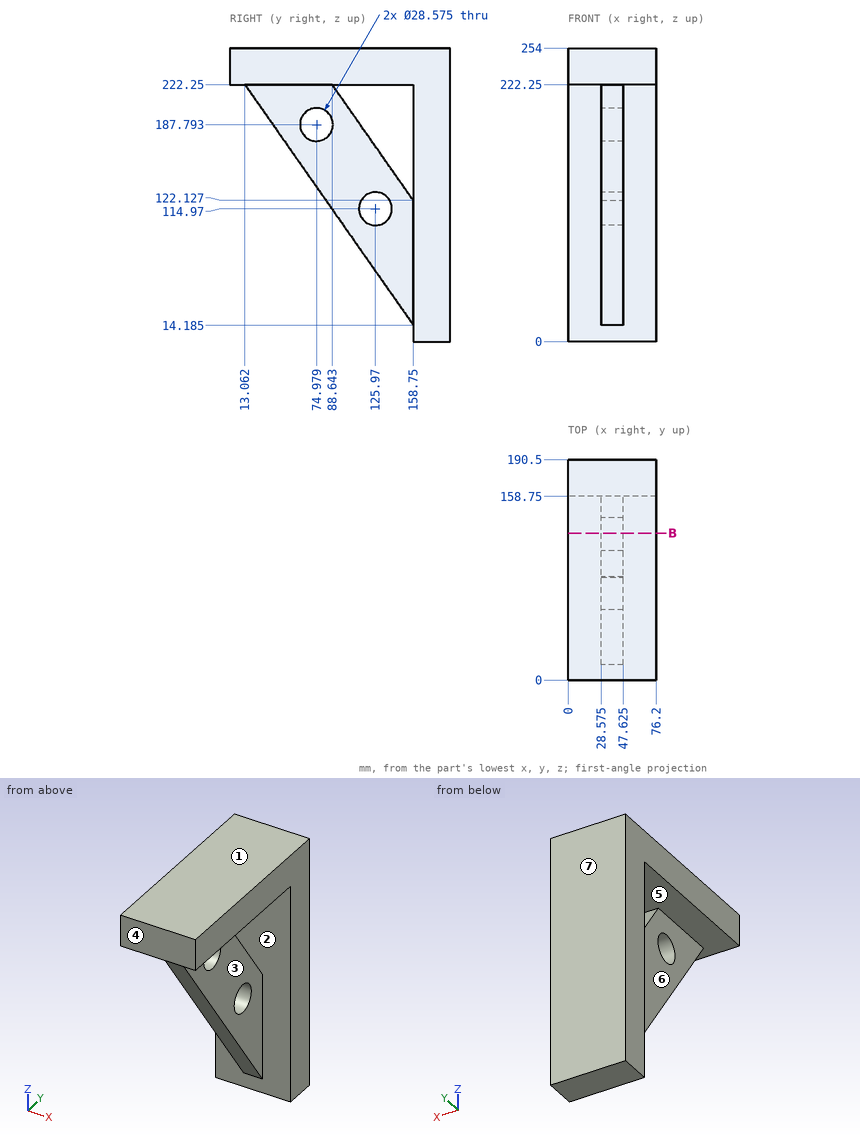
Geometry check sheet. Reference: drawing and pictorial views, mm from the part's lowest x, y, z. A direction names the side the tool comes from. Round coordinates to 2 decimals unless told otherwise and drop trailing zeros. Answer as a JSON object with one key per item and string values.
Q1. Scan lines: line 1 (Y direction, x = 12.5, z = 112.5); line 2 (X direction, y = 116.5, z = 84.5) (1 decimal); line 3 (Z direction, x = 63.5, y = 82.5). Record each from-to range of solid material in increasing order. Write a range as from..to.
Data:
{"line 1": "y = 158.75..190.5", "line 2": "x = 28.6..47.6", "line 3": "z = 222.25..254"}
Q2. Draft check along Y on the marked faces 4, 5, 6 and 7. Enter one of: pulls with the +Y half, pulls with the -Y half, needs draft (parallel to the pull), parting line crosses it, or undercut.
Data:
{"face 4": "pulls with the -Y half", "face 5": "undercut", "face 6": "needs draft", "face 7": "pulls with the +Y half"}
Q3. Section check B-B (y = 127). State how many separate pieces and enclosed holes the cut face has, then the cut area to 3 significant figures.
Data:
{"separate pieces": "3", "enclosed holes": "0", "area": "3,930 mm2"}
Q4. Access from +Z, -Z, +X, -X, +Y, -Y to the whole of each face (thin tool, end or side, straight path). Record for the marked faces 1, 2 and 3.
Data:
{"face 1": "+Z, +X, -X, +Y, -Y", "face 2": "none", "face 3": "-Z, +X, -Y"}
Q5. Go/stop test with flat-tipped pins: P1, Ø23, axis at x = 21, z = 69, coming from the -Y side; P2, Ø10, axis at x = 35, y = 110, coming from the -Z side (1 decimal); P3, Ø2, axis at y = 165.5, z = 196.5, coming from the -X side; P4, Ø10, axis at y = 91.5, z = 144, coming from the +X side (1 decimal). Record where each tip stops, or that it passes through.
Data:
{"P1": "stops at y = 114.31", "P2": "stops at z = 76.7", "P3": "stops at x = 0", "P4": "stops at x = 47.6"}
